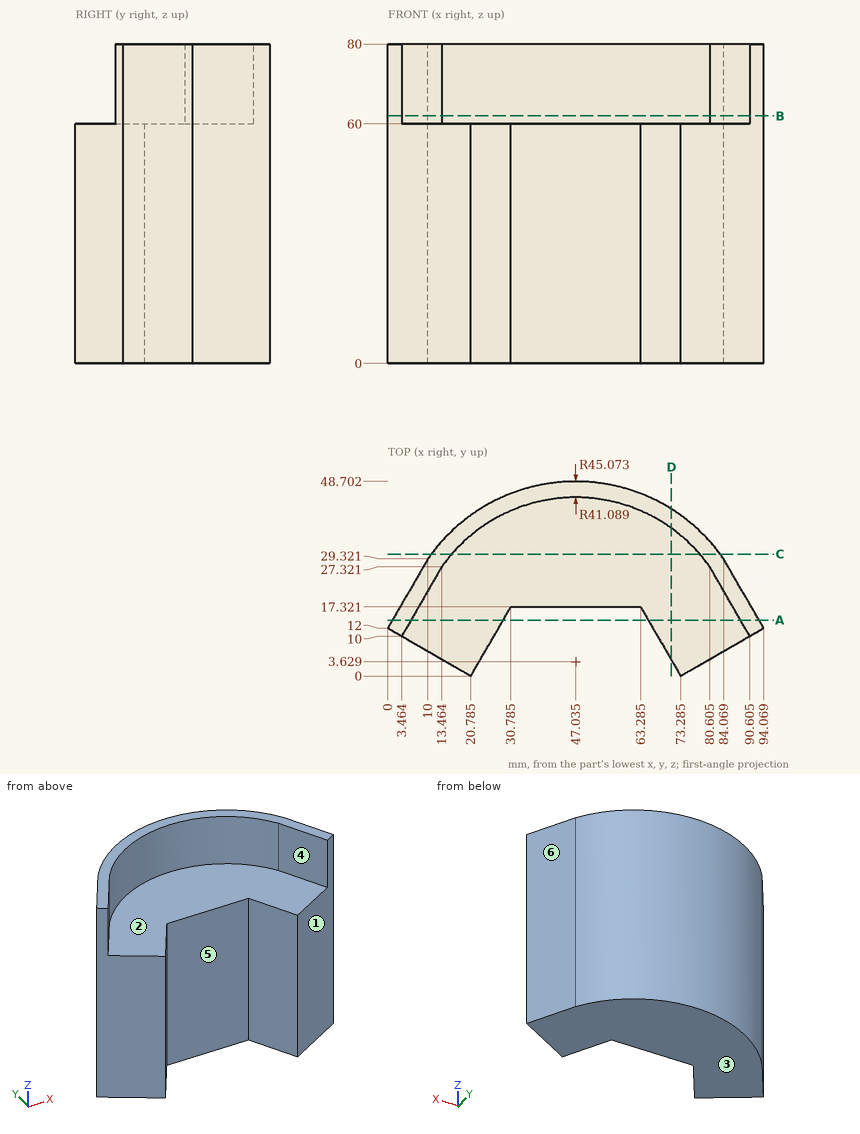
Could you check a few things on this drawing? It's one solid part, dimensions in mm from its lowest x, y, z. A direction names the side the tool comes from. Round coordinates to 2 decimals unless told otherwise and drop trailing zeros. Loops run counter-clockwise (first coordinate to the right, second up) from the corner with the lowest first, then second, coordinate; pieces in that order, holes last. Notation, with made-up numbers: M 32.5,86.25 L 40.5,86.25 A25 ccw 40.5,115.25 Z; hole C 38,59 d9. An arc over 180 degrees is marked long. Write each question's results on one line, items separated by ' | '. Start each with the question number.
(1) Will these pins go through, and if not, where does the flat tip stop? P1, Ø10, axis at x = 37, z = 42.5, coming from the +Y side; P2, Ø2, axis at x = 67.5, z = 19, coming from the -Y side (1 decimal); P3, Ø2, axis at x = 50.5, z = 38, coming from the -Y side.
(2) Thinking about a two-plate mould opening in X: for the marked faces 1, 2 and 3, which applies, pulls with the +X half, pulls with the -X half, needs draft (parallel to the pull), parting line crosses it, or undercut?
(3) I want a section at B-B (z = 62). Please give me the cut outline in (x, y) (1 decimal).
(4) I want a section at C-C (y = 30.5). Please give me the cut outline in (x, z).
(5) On a 3-axis mill with a long thin cutter (end or side, diameter ignored), from which of +Z, -Z, +X, -X, +Y, -Y can I reach the whole of each face in a straight line? I mean the marked faces 4, 5 and 6. Say none if no direction works.
(6) I want a section at A-A (y = 14). Please give me the cut outline in (x, z) (1 decimal).
(7) If I drill on probe 1 along X at (y, z) = (4.5, 54.5) (1 decimal); probe 2 along Z at (x, y) = (28, 35.5); probe 3 along X at (y, z) = (9, 55.5) (1 decimal), over which ranges is the centre line in solid material (lowest first)? Write a range as from..to.
(8) I want a section at D-D (x = 71). Please give me the cut outline in (y, z) (1 decimal), then the cut area to 3 significant figures.
Solved:
1) P1: stops at y = 48.42 | P2: stops at y = 8.3 | P3: stops at y = 17.32
2) face 1: pulls with the +X half | face 2: undercut | face 3: needs draft
3) outline: M 0,12 L 3.5,10 L 13.5,27.3 A41.1 cw 80.6,27.3 L 90.6,10 L 94.1,12 L 84.1,29.3 A45.1 ccw 10,29.3 Z
4) outline: M 10.85,0 L 83.22,0 L 83.22,80 L 78.12,80 L 78.12,60 L 15.95,60 L 15.95,80 L 10.85,80 Z
5) face 4: +Z, -Y | face 5: +Z, -Z, -Y | face 6: +Z, -Z, +X, +Y
6) outline: M 1.2,0 L 28.9,0 L 28.9,60 L 5.8,60 L 5.8,80 L 1.2,80 Z; M 65.2,0 L 92.9,0 L 92.9,80 L 88.3,80 L 88.3,60 L 65.2,60 Z
7) probe 1: x = 13..23.4, 70.7..81.1 | probe 2: z = 0..60 | probe 3: x = 5.2..26, 68.1..88.9
8) outline: M 4,0 L 41.8,0 L 41.8,80 L 37,80 L 37,60 L 4,60 Z | area: 2,370 mm²
